Work out the finished part from the listing and answer in its coordinate system (mm). A direction names the side the tool comes from. Give positions to 0.01 mm unless a question says otherwise; leave off trailing zeros. Write each loop counter-clockwise with the first axis right and the second up, starting at its lowest first coordinate (ties: lowest second). Pieces come first, ordered by that corner, then holes. Notation, with made-up numbers: (8, 27.5) - (17, 27.5) arc R10 cw to (17, 32.5) - close; hole circle Ø11 at (60, 1). An arc over 180 degrees is marked (long way). Write item = value, one per line.
from build123d import *

# Parameters (mm, degrees)
SKETCH1_R           = 60
BOSS_EXTRUDE1_DEPTH = 10
BOSS_EXTRUDE2_START = 20
BOSS_EXTRUDE2_DEPTH = 10


with BuildPart() as part:
    # Sketch1 → Boss-Extrude1 (new body)
    with BuildSketch(Plane(origin=(0, 0, 0), x_dir=(1, 0, 0), z_dir=(0, 1, 0))):
        with Locations(Location((0, 0, 0), (0, 0, 270))):
            Circle(SKETCH1_R)
    extrude(amount=-BOSS_EXTRUDE1_DEPTH)

    # Sketch2 → Boss-Extrude2 (add)
    with BuildSketch(Plane(origin=(0, 0, 0), x_dir=(0, 0, -1), z_dir=(1, 0, 0)).offset(BOSS_EXTRUDE2_START)):
        with BuildLine():
            Line((0, 0), (50, 0))
            Line((50, 0), (50, 50))
            ThreePointArc((50, 50), (0, 100), (-50, 50))
            Line((-50, 50), (-50, 0))
            Line((-50, 0), (0, 0))
        make_face()
    boss_extrude2 = extrude(amount=BOSS_EXTRUDE2_DEPTH)

    # Mirror1: Boss-Extrude2 across plane
    add(boss_extrude2.mirror(Plane(origin=(0, 0, 0), x_dir=(0, 0, 1), z_dir=(1, 0, 0))))


solid = part.part
1. Find section D-D, the plane y = 75. Give the vertices of the cut face in (x, z), then the cut area to 3 significant figures.
Solution:
outline = (-30, -43.3) - (-20, -43.3) - (-20, 43.3) - (-30, 43.3) - close; (20, -43.3) - (30, -43.3) - (30, 43.3) - (20, 43.3) - close
area = 1,730 mm^2
2. Find section C-C, the plane x = 0. Give the vertices of the cut face in (y, z).
Solution:
outline = (-10, -60) - (0, -60) - (0, 60) - (-10, 60) - close
3. Straight lines are drawn through the part: line 1 (X direction, y = 14.5, z = 6); line 2 (Y direction, x = -3.5, z = -37); line 3 (X direction, y = -3, z = 50). For each, find the intervals that lie inside material, in ascending order.
Solution:
line_1 = -30 to -20, 20 to 30
line_2 = -10 to 0
line_3 = -33.17 to 33.17
4. Find section B-B, the plane z = 0. Give the vertices of the cut face in (x, y), then the cut area to 3 significant figures.
Solution:
outline = (-60, -10) - (60, -10) - (60, 0) - (30, 0) - (30, 100) - (20, 100) - (20, 0) - (-20, 0) - (-20, 100) - (-30, 100) - (-30, 0) - (-60, 0) - close
area = 3,200 mm^2
5. Find section A-A, the plane y = 47. Give the vertices of the cut face in (x, z), then the cut area to 3 significant figures.
Solution:
outline = (-30, -50) - (-20, -50) - (-20, 50) - (-30, 50) - close; (20, -50) - (30, -50) - (30, 50) - (20, 50) - close
area = 2,000 mm^2
6. Given pin 1 (6 mm diameter, centred on y = 31, z = -40.5, fed in from +X); pin 2 (3 mm diameter, centred on x = -20.5, y = 45.5, fed in from -Z); pin 3 (4 mm diameter, centred on y = 58.5, z = 13, fed in from -X), each flat-ended and moving along its own axis, determine where each tip first touches the part or whether it passes through.
Solution:
pin_1 = 30
pin_2 = -50
pin_3 = -30
7. A tool of negligible diameter and unlimited length cuts with its end or side. For faces 1 (the flat face through (25, 25, 50)), 2 (the flat face through (30, 51, 1)), 3 (the flat face through (-30, 51, 1)), 4 (the flat face through (-25, 25, -50)), 5 (the flat face through (20, 51, 1)), from which of +Z, -Z, +X, -X, +Y, -Y can it reach the whole face along a straight path? Write none if from no direction.
Solution:
face_1 = +Z, +X, -X, +Y
face_2 = +Z, -Z, +X, +Y
face_3 = +Z, -Z, -X, +Y
face_4 = -Z, +X, -X, +Y
face_5 = +Z, -Z, +Y
